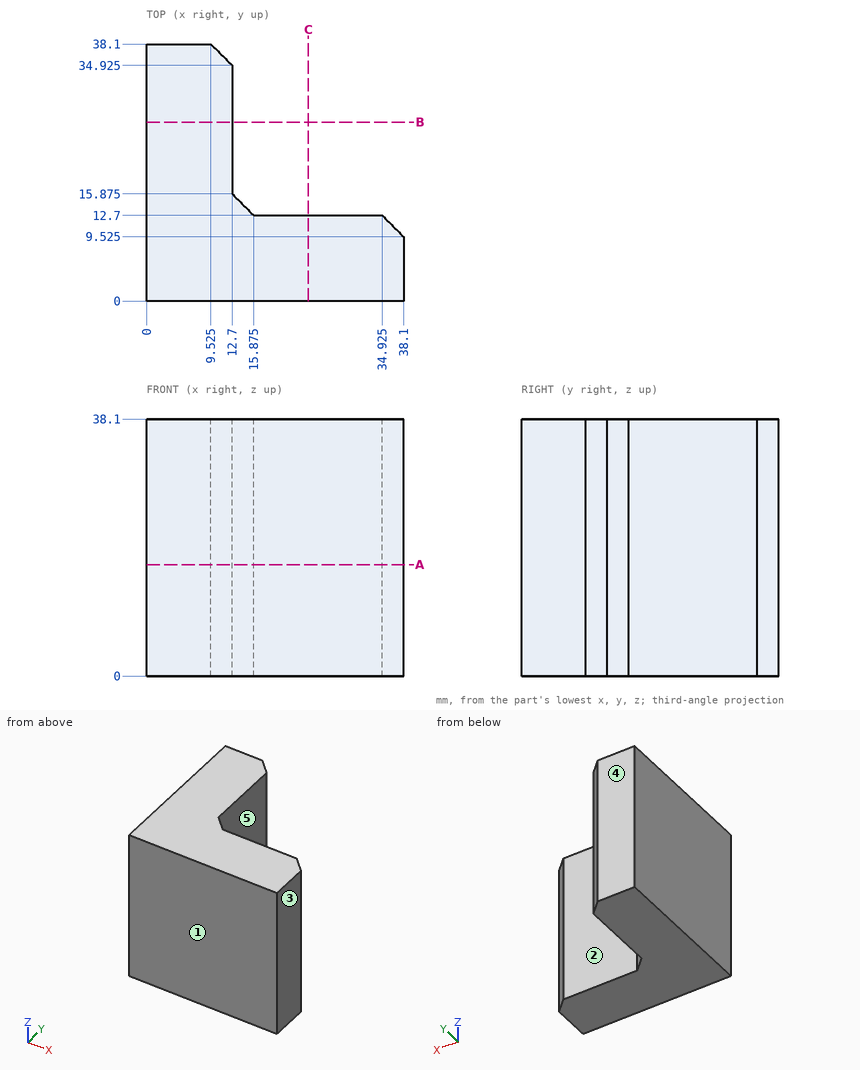
Check sheet for the drawn part. Datum: minimum x, y, z corner. Units: mm. A direction names the side the tool comes from. Give positions to 0.01 mm unless a question says otherwise; leave off trailing zeros. Write each loop counter-clockwise with the first axis right and the second up, starting at its lowest first coordinate (ties: lowest second). Pieces come first, ordered by that corner, then holes. Notation, with made-up numbers: (-1, 39.25) - (17, 39.25) arc R26 ccw to (17, 78.25) - close; hole circle Ø1 at (-9, 86.25). An arc over 180 degrees is marked (long way). Put each result on its own line as item: value.
1. Go/stop test with flat-tipped pins: pin 1 (1 mm diameter, centred on x = 13, z = 10.5, fed in from +Y) (3 decimals); pin 2 (21 mm diameter, centred on x = 29, z = 17.5, fed in from +Y); pin 3 (8 mm diameter, centred on y = 15, z = 32.5, fed in from +X) (3 decimals). Record where each tip stops, or that it passes through.
Ans:
pin 1: stops at y = 35.125
pin 2: stops at y = 12.7
pin 3: stops at x = 36.625
2. Sectioned sample at A-A, the plane z = 16.5. Enter the section's corners in (x, y) (3 decimals).
Ans:
outline: (0, 0) - (38.1, 0) - (38.1, 9.525) - (34.925, 12.7) - (15.875, 12.7) - (12.7, 15.875) - (12.7, 34.925) - (9.525, 38.1) - (0, 38.1) - close
3. Sectioned sample at B-B, the plane y = 26.5. Enter the section's corners in (x, z).
Ans:
outline: (0, 0) - (12.7, 0) - (12.7, 38.1) - (0, 38.1) - close
4. Thickness scan on line 1 (X direction, y = 31.5, z = 10); line 2 (X direction, y = 15, z = 30) (3 decimals). Record the ranges inside material, lowest first.
Ans:
line 1: x = 0 to 12.7
line 2: x = 0 to 13.575
5. Set-up check for the marked faces 4 and 5: record each of +Z, -Z, +X, -X, +Y, -Y from which the full face is reachable in a straight line by a thin tool's end or side.
Ans:
face 4: +Z, -Z, +X, -X, +Y
face 5: +Z, -Z, +X, +Y
6. Draft check along Y on the marked faces 1, 2 and 3. Enter one of: +Y half, -Y half, draft (parallel to the pull), parting line (faces both ways), or undercut.
Ans:
face 1: -Y half
face 2: +Y half
face 3: draft
